The figure shows three views and two pictorial views of one solid part (mm, origin at its lowest corner). Answer the questions. Give positions to 0.01 mm unless a question says otherwise; leave off trailing zeros. Loops run counter-clockwise (first coordinate to the right, second up) from the corner with the lowest first, then second, coordinate; pieces in that order, holes last. Notation, with made-up numbers: (81, 74.5) - (123, 74.5) arc R13 cw to (123, 80.5) - close; hole circle Ø11 at (46.25, 40.25). An arc over 180 degrees is marked (long way). Write item = value, one per line.
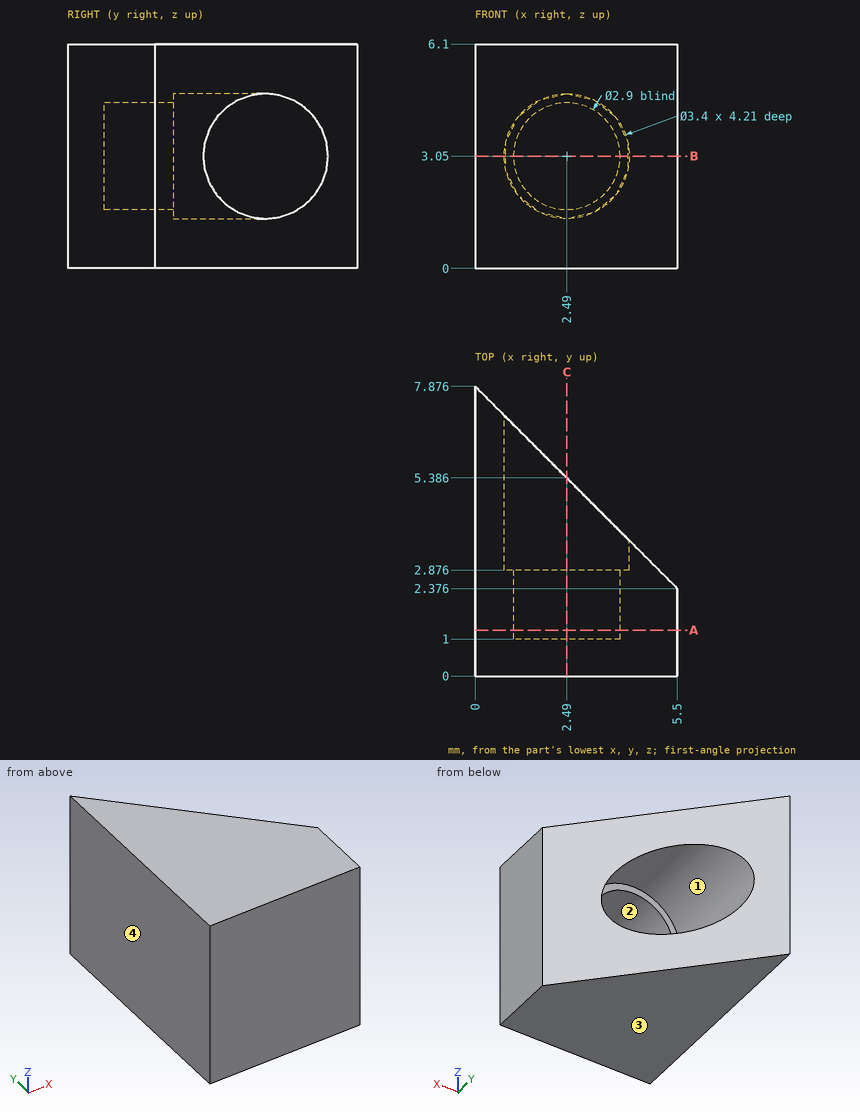
1) A cutting plane is placed at B-B on z = 3.05. Determine the outline of the cut face in (x, y), then the cut area to 3 significant figures.
Output:
outline = (0, 0) - (5.5, 0) - (5.5, 2.38) - (4.19, 3.69) - (4.19, 2.88) - (3.94, 2.88) - (3.94, 1) - (1.04, 1) - (1.04, 2.88) - (0.79, 2.88) - (0.79, 7.09) - (0, 7.88) - close
area = 14.2 mm²
2) A cutting plane is placed at A-A on y = 1.25. Determine the outline of the cut face in (x, z).
Output:
outline = (0, 0) - (5.5, 0) - (5.5, 6.1) - (0, 6.1) - close; hole circle Ø2.9 at (2.49, 3.05)
3) A cutting plane is placed at C-C on x = 2.49. Determine the outline of the cut face in (y, z).
Output:
outline = (0, 0) - (5.39, 0) - (5.39, 1.35) - (2.88, 1.35) - (2.88, 1.6) - (1, 1.6) - (1, 4.5) - (2.88, 4.5) - (2.88, 4.75) - (5.39, 4.75) - (5.39, 6.1) - (0, 6.1) - close
4) The mould has two halves that part along Z. Classify the marked faces 1, 2, 3 and 4: pulls with the +Z half, pulls with the -Z half, needs draft (parallel to the pull), parting line crosses it, or undercut.
Output:
face_1 = undercut
face_2 = undercut
face_3 = pulls with the -Z half
face_4 = needs draft
5) Each of these flat-tipped pins is pushed along its axis until it touches: P1, Ø2, axis at y = 4, z = 3, coming from the +X side (1 decimal); P2, Ø2.5, axis at x = 2.5, z = 3, coming from the +Y side. Where does it stop, or does it pass through?
Output:
P1 = 4.9
P2 = 1
6) Find the intervals of material crossed by probe 1 along X at (y, z) = (2.2, 3.05); probe 2 along Z at (x, y) = (2.49, 1.45); probe 3 along X at (y, z) = (6.2, 3.05), in increasing order.
Output:
probe_1 = 0 to 1.04, 3.94 to 5.5
probe_2 = 0 to 1.6, 4.5 to 6.1
probe_3 = 0 to 0.79
